Can you work these out from the model? Positions are in its coordinate system, mm. Face numbers are marked on the shaded views. A direction names the side the tool comes from. Coordinates: 2 decimals unless noted, no trailing zeros. Order: outer loops, then holes, each group sorted by start corner. A loop starts at its lowest first (then second) coordinate and runs counter-clockwise, first axis right, second up.
```python
from build123d import *
from build123d.topology import SkipClean

# Parameters (mm, degrees)
SKETCH_1_R                         = 50
EXTRUDE_18_DEPTH                   = 13
EXTRUDE_18_2_DEPTH                 = 13
SKETCH_1_28_W                      = 300
SKETCH_1_28_H                      = 100
EXTRUDE_21_DEPTH                   = 15
SKETCH_1_30_R                      = 5
EXTRUDE_22_DEPTH                   = 70
SKETCH_1_31_R                      = 50
CUT_EXTRUDE_2_DEPTH                = 41
EXTRUDE_23_DEPTH                   = 18
EXTRUDE_23_DEPTH_BACK              = 1
SKETCH_1_32_R                      = 50
CUT_EXTRUDE_5_DEPTH                = 130
CUT_EXTRUDE_5_DEPTH_BACK           = 69
SKETCH_1_35_R                      = 3.175
SKETCH_1_36_R                      = 50
CUT_EXTRUDE_6_DEPTH                = 34
EXTRUDE_24_DEPTH                   = 18
EXTRUDE_24_DEPTH_BACK              = 3
SKETCH_1_37_R                      = 50
CUT_EXTRUDE_7_DEPTH                = 87
CUT_EXTRUDE_7_DEPTH_BACK           = 98
SKETCH_1_41_R                      = 3.175
THE_EXTENDED_SHAFT_CONNECTER_DEPTH = 36
SKETCH_3_R                         = 1.5875
CUT_EXTRUDE_8_DEPTH                = 31
SCREW_HOLES2_REACH                 = 372.675
SCREW_HOLES2_END_RADIUS            = 6.25
SKETCH_5_R                         = 1.5875


with BuildPart() as part:
    # Sketch 1 → Extrude 18 (new body)
    with BuildSketch(Plane.XY):
        with Locations(Location((0, 50, 0), (0, 0, 180))):
            Circle(SKETCH_1_R)
    extrude(amount=EXTRUDE_18_DEPTH)



with BuildPart() as body_2:
    # Sketch 1 → Extrude 18 2 (new body)
    with BuildSketch(Plane.XY):
        with Locations(Location((-300, 50, 0), (0, 0, 180))):
            Circle(SKETCH_1_R)
    extrude(amount=EXTRUDE_18_2_DEPTH)


with BuildPart() as part_1:
    add(part.part)

    add(body_2.part)  # Extrude 21 merges body 2
    # Sketch 1_28 → Extrude 21 (add)
    with BuildSketch(Plane.XY):
        with Locations((-150, 50)):
            Rectangle(SKETCH_1_28_W, SKETCH_1_28_H)
    extrude(amount=EXTRUDE_21_DEPTH)

    # Sketch 1_30 → Extrude 22 (add)
    with BuildSketch(Plane.XY):
        with Locations((-150, 50)):
            Circle(SKETCH_1_30_R)
    extrude(amount=EXTRUDE_22_DEPTH)

    # Sketch 1_31 → Cut-Extrude 2 (cut)
    with BuildSketch(Plane.XY):
        with Locations((-300, 50)):
            Circle(SKETCH_1_31_R)
    extrude(amount=CUT_EXTRUDE_2_DEPTH, mode=Mode.SUBTRACT)

    # Sketch 1_32 → Extrude 23 (add, two sides: drawn at the far end of the back side and taken through both)
    with BuildSketch(Plane.XY.offset(-EXTRUDE_23_DEPTH_BACK)):
        with Locations((-300, 50)):
            Circle(SKETCH_1_32_R)
    extrude(amount=EXTRUDE_23_DEPTH + EXTRUDE_23_DEPTH_BACK)

    # Sketch 1_35 → Cut-Extrude 5 (cut, two sides: drawn at the far end of the back side and taken through both)
    with BuildSketch(Plane.XY.offset(-CUT_EXTRUDE_5_DEPTH_BACK)):
        with Locations((-261.469660941, 50)):
            Circle(SKETCH_1_35_R)
    extrude(amount=CUT_EXTRUDE_5_DEPTH + CUT_EXTRUDE_5_DEPTH_BACK, mode=Mode.SUBTRACT)

    # Sketch 1_36 → Cut-Extrude 6 (cut)
    with BuildSketch(Plane.XY):
        with Locations((0, 50)):
            Circle(SKETCH_1_36_R)
    extrude(amount=CUT_EXTRUDE_6_DEPTH, mode=Mode.SUBTRACT)

    # Sketch 1_37 → Extrude 24 (add, two sides: drawn at the far end of the back side and taken through both)
    with BuildSketch(Plane.XY.offset(-EXTRUDE_24_DEPTH_BACK)):
        with Locations((0, 50)):
            Circle(SKETCH_1_37_R)
    extrude(amount=EXTRUDE_24_DEPTH + EXTRUDE_24_DEPTH_BACK)

    # Sketch 1_41 → Cut-Extrude 7 (cut, two sides: drawn at the far end of the back side and taken through both)
    with BuildSketch(Plane.XY.offset(-CUT_EXTRUDE_7_DEPTH_BACK)):
        with Locations((-272.75493597, 77.24506403)):
            Circle(SKETCH_1_41_R)
        with BuildLine():
            ThreePointArc((-296.825, 88.530339059), (-297.75493597, 90.77540309), (-300, 91.705339059))
            Line((-300, 91.705339059), (-300, 85.355339059))
            ThreePointArc((-300, 85.355339059), (-297.75493597, 86.285275029), (-296.825, 88.530339059))
        make_face()
        with BuildLine():
            Line((-300, 85.355339059), (-300, 91.705339059))
            ThreePointArc((-300, 91.705339059), (-303.175, 88.530339059), (-300, 85.355339059))
        make_face()
        with Locations((-327.24506403, 77.24506403)):
            Circle(SKETCH_1_41_R)
        with Locations((-338.530339059, 50)):
            Circle(SKETCH_1_41_R)
        with BuildLine():
            ThreePointArc((-325, 25), (-329.490128061, 25), (-329.490128061, 20.509871939))
            Line((-329.490128061, 20.509871939), (-325, 25))
        make_face()
        with BuildLine():
            Line((-325, 25), (-329.490128061, 20.509871939))
            ThreePointArc((-329.490128061, 20.509871939), (-326.030044133, 19.821618454), (-324.07006403, 22.75493597))
            ThreePointArc((-324.07006403, 22.75493597), (-324.311746515, 23.969955867), (-325, 25))
        make_face()
        with BuildLine():
            ThreePointArc((-300, 14.644660941), (-303.175, 11.469660941), (-300, 8.294660941))
            Line((-300, 8.294660941), (-300, 14.644660941))
        make_face()
        with BuildLine():
            Line((-300, 14.644660941), (-300, 8.294660941))
            ThreePointArc((-300, 8.294660941), (-297.75493597, 9.22459691), (-296.825, 11.469660941))
            ThreePointArc((-296.825, 11.469660941), (-297.75493597, 13.714724971), (-300, 14.644660941))
        make_face()
        with Locations((-272.75493597, 22.75493597)):
            Circle(SKETCH_1_41_R)
        with BuildLine():
            ThreePointArc((-264.644660941, 50), (-261.469660941, 46.825), (-258.294660941, 50))
            Line((-258.294660941, 50), (-264.644660941, 50))
        make_face()
        with BuildLine():
            Line((-264.644660941, 50), (-258.294660941, 50))
            ThreePointArc((-258.294660941, 50), (-261.469660941, 53.175), (-264.644660941, 50))
        make_face()
        with Locations((-27.24506403, 22.75493597)):
            Circle(SKETCH_1_41_R)
        with Locations((-38.530339059, 50)):
            Circle(SKETCH_1_41_R)
        with Locations((-27.24506403, 77.24506403)):
            Circle(SKETCH_1_41_R)
        with BuildLine():
            ThreePointArc((3.175, 88.530339059), (2.24506403, 90.77540309), (0, 91.705339059))
            Line((0, 91.705339059), (0, 85.355339059))
            ThreePointArc((0, 85.355339059), (2.24506403, 86.285275029), (3.175, 88.530339059))
        make_face()
        with BuildLine():
            Line((0, 85.355339059), (0, 91.705339059))
            ThreePointArc((0, 91.705339059), (-3.175, 88.530339059), (0, 85.355339059))
        make_face()
        with Locations((27.24506403, 77.24506403)):
            Circle(SKETCH_1_41_R)
        with Locations((27.24506403, 22.75493597)):
            Circle(SKETCH_1_41_R)
        with Locations((38.530339059, 50)):
            Circle(SKETCH_1_41_R)
        with BuildLine():
            ThreePointArc((0, 14.644660941), (-3.175, 11.469660941), (0, 8.294660941))
            Line((0, 8.294660941), (0, 14.644660941))
        make_face()
        with BuildLine():
            Line((0, 14.644660941), (0, 8.294660941))
            ThreePointArc((0, 8.294660941), (2.24506403, 9.22459691), (3.175, 11.469660941))
            ThreePointArc((3.175, 11.469660941), (2.24506403, 13.714724971), (0, 14.644660941))
        make_face()
    extrude(amount=CUT_EXTRUDE_7_DEPTH + CUT_EXTRUDE_7_DEPTH_BACK, mode=Mode.SUBTRACT)

    # Sketch 1_43 → the extended shaft connecter (add)
    with BuildSketch(Plane.XY):
        with BuildLine():
            Line((0, 43.75), (0, 40.475))
            ThreePointArc((0, 40.475), (6.735192091, 43.264807909), (9.525, 50))
            ThreePointArc((9.525, 50), (6.735192091, 56.735192091), (0, 59.525))
            Line((0, 59.525), (0, 56.25))
            ThreePointArc((0, 56.25), (3.642600233, 55.078775791), (5.919983963, 52.004068333))
            Line((5.919983963, 52.004068333), (6.25, 52.004068333))
            Line((6.25, 52.004068333), (8.25, 52.004068333))
            Line((8.25, 52.004068333), (8.25, 50))
            Line((8.25, 50), (8.25, 47.995931667))
            Line((8.25, 47.995931667), (6.25, 47.995931667))
            Line((6.25, 47.995931667), (5.919983963, 47.995931667))
            ThreePointArc((5.919983963, 47.995931667), (3.642600233, 44.921224209), (0, 43.75))
        make_face()
        with BuildLine():
            ThreePointArc((0, 59.525), (-9.525, 50), (0, 40.475))
            Line((0, 40.475), (0, 43.75))
            ThreePointArc((0, 43.75), (-6.25, 50), (0, 56.25))
            Line((0, 56.25), (0, 59.525))
        make_face()
    extrude(amount=-THE_EXTENDED_SHAFT_CONNECTER_DEPTH)

    # Sketch 3 → Cut-Extrude 8 (cut)
    with BuildSketch(Plane(origin=(0, 0, 0), x_dir=(0, 0, -1), z_dir=(1, 0, 0))):
        with Locations((32, 50)):
            Circle(SKETCH_3_R)
        with Locations((25, 50)):
            Circle(SKETCH_3_R)
    extrude(amount=-CUT_EXTRUDE_8_DEPTH, mode=Mode.SUBTRACT)

    # screw_holes2: up to this cylinder (the profile starts outside it)
    with SkipClean():  # the faces are left unmerged after this step: merging them gives an invalid solid
        screw_holes2_end = Plane(origin=(0, 50, -28.5), z_dir=(0, 0, 1)) * Cylinder(SCREW_HOLES2_END_RADIUS, 765.85, mode=Mode.PRIVATE)
        # Sketch 5 → screw_holes2 (cut, up to the surface)
        with BuildSketch(Plane(origin=(0, 0, 0), x_dir=(1, 0, 0), z_dir=(0, 1, 0)), mode=Mode.PRIVATE) as screw_holes2_sk1:
            with Locations(Location((0, 32, 0), (0, 0, 90))):
                Circle(SKETCH_5_R)
        screw_holes2_tool1 = extrude(screw_holes2_sk1.sketch, amount=SCREW_HOLES2_REACH, mode=Mode.PRIVATE) - screw_holes2_end
        add(screw_holes2_tool1.solids().sort_by_distance((0, 0, -32))[0], mode=Mode.SUBTRACT)
        # Sketch 5 → screw_holes2 (cut, up to the surface)
        with BuildSketch(Plane(origin=(0, 0, 0), x_dir=(1, 0, 0), z_dir=(0, 1, 0)), mode=Mode.PRIVATE) as screw_holes2_sk2:
            with Locations(Location((0, 25, 0), (0, 0, 90))):
                Circle(SKETCH_5_R)
        screw_holes2_tool2 = extrude(screw_holes2_sk2.sketch, amount=SCREW_HOLES2_REACH, mode=Mode.PRIVATE) - screw_holes2_end
        add(screw_holes2_tool2.solids().sort_by_distance((0, 0, -25))[0], mode=Mode.SUBTRACT)


solid = part_1.part
```
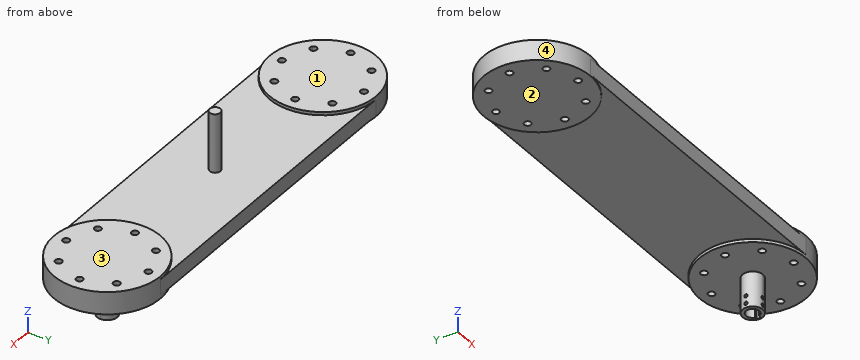
1. Thinking about a two-plate mould opening in X: for the marked faces 3 and 4, which applies, pulls with the +X half, pulls with the -X half, needs draft (parallel to the pull), parting line crosses it, or undercut?
Completed:
face 3: needs draft
face 4: undercut
2. I'm going to push flat-ended pins straight in: pin 1 (4.5 mm diameter, centred on y = 50.5, z = -13, fed in from -X) (3 decimals); pin 2 (6 mm diameter, centred on x = -222.5, y = 82, fed in from -Z); pin 3 (12 mm diameter, centred on x = -306.5, z = 8.5, fed in from -Y). Where does each tip first touch, or does it pass through?
Completed:
pin 1: stops at x = -9.525
pin 2: stops at z = 0
pin 3: stops at y = 0
3. Imagine slicing it at B-B on x = -150. Please give me the cut outline in (y, z).
Completed:
outline: (0, 0) - (100, 0) - (100, 15) - (55, 15) - (55, 70) - (45, 70) - (45, 15) - (0, 15) - close
4. Imagine slicing it at C-C on y = 33. Please give me the cut outline in (x, z).
Completed:
outline: (-347.02, -1) - (-252.98, -1) - (-252.98, 0) - (-47.02, 0) - (-47.02, -3) - (47.02, -3) - (47.02, 18) - (-47.02, 18) - (-47.02, 15) - (-252.98, 15) - (-252.98, 18) - (-347.02, 18) - close
5. On a 3-axis mill with a long thin cutter (end or side, diameter ignored), from which of +Z, -Z, +X, -X, +Y, -Y can I reach the whole of each face in a straight line? I mean the marked faces 1 and 2. Say none if no direction works.
Completed:
face 1: +Z, -X, +Y, -Y
face 2: -Z, -X, +Y, -Y
6. Imagine slicing it at A-A on z = -10. Please give me the cut outline in (x, y) (3 decimals).
Completed:
outline: circle Ø19.05 at (0, 50); hole (5.92, 47.996) - (8.25, 47.996) - (8.25, 52.004) - (5.92, 52.004) arc R6.25 ccw (long way) to start
7. Imagine slicing it at D-D on x = -290.5. Please give me the cut outline in (y, z).
Completed:
outline: (0, 0) - (0.91, 0) - (0.91, -1) - (99.09, -1) - (99.09, 0) - (100, 0) - (100, 15) - (99.09, 15) - (99.09, 18) - (0.91, 18) - (0.91, 15) - (0, 15) - close
8. Please list where these lines run through material, in increasing order: probe 1 along Z at (x, y) = (-7.5, 16); probe 2 along Z at (x, y) = (-139, 10.5); probe 3 along Y at (x, z) = (-7, -32).
Completed:
probe 1: z = -3 to 18
probe 2: z = 0 to 15
probe 3: y = 43.54 to 48.41, 51.59 to 56.46
